Build history of the part. All positions in model axes, mm. A direction names the side the tool comes from. Give positions to 0.01 mm unless a question says otherwise; leave off trailing zeros. Order: outer loops, then holes, each group sorted by start corner. A loop starts at its lowest first (then second) coordinate and runs counter-clockwise, first axis right, second up. Notation, with made-up numbers: (38, -39.5) - (93, -39.5) arc R15 ccw to (93, -21.5) - close; hole circle Ø3 at (84, 55.5). An arc over 180 degrees is marked (long way). Use a Markdown table: item, result. Add a question column.
(1) Wall check: line 1 (Y direction, x = -8.5, z = 0); line 2 (Y direction, x = -14.55, z = 0); line 3 (Z direction, x = -7, y = -3.5). Give the ranges that are in metal, low to high.
(2) Slice it at A-A (y = 0). Write the cut outline in (x, z), then the cut area to 3 significant figures.
(3) Mould opens along Y. For faces 3 (the face through (-14.26, -15.62, -3.47)), 4 (the face through (0, -14, 14)), 5 (the face through (-6.844, -16.856, 8.767)), 6 (the face through (-7.409, -21.317, -2.799)) say: +Y half, -Y half, draft (parallel to the pull), parting line (faces both ways), or undercut.
(4) Slice it at C-C (x = -5.5). Write the cut outline in (y, z).
(5) Flat gauge pins, fed straight in: pin 1 (1.5 mm diameter, centred on x = -5.5, z = -14, fed in from -Y); pin 2 (5 mm diameter, centred on x = -5.5, z = 12.5, fed in from -Y); pin 3 (8 mm diameter, centred on y = 6.5, z = -7.5, fed in from -X); pin 4 (3 mm diameter, centred on x = -12.5, y = 5, fed in from +Z). Where does each tip first touch, or does it go through?
(6) Which spindle directions (+Z, -Z, +X, -X, +Y, -Y) get a long thin tool onto all of the face, cutting with end or side? Do faces 1 (the face through (-13.5, -13, -10)), 2 (the face through (-15, -11, 12)). Say none if no direction does.
Autodesk Inventor part; units mm, degrees
ref_plane "YZ Plane" through (0, 0, 0) normal (1, 0, 0) x (0, 1, 0)
ref_plane "XZ Plane" through (0, 0, 0) normal (0, 1, 0) x (-1, 0, 0)
ref_plane "XY Plane" through (0, 0, 0) normal (0, 0, 1) x (1, 0, 0)
sketch "Sketch1" plane through (0, 0, 0) normal (0, 1, 0) x (-1, 0, 0)
  line L0 (0, 0) -> (15, 0)
  line L1 (15, 16) -> (15, 21.5)
  line L2 (15, 21.5) -> (0, 21.5)
  line L3 (0, 21.5) -> (0, 19)
  line L4 (0, 19) -> (13.5, 19)
  line L5 (13.5, 19) -> (13.5, 16)
  line L6 (13.5, 16) -> (15, 16)
  dimension "d0" = 38
  dimension "d1" = 2.5
  dimension "d2" = 15
  dimension "d3" = 1.5
  dimension "d6" = 32
revolve "Revolution1" add sketch "Sketch1" angle 360 about axis through (0, 0, 0) along (-1, 0, 0)
chamfer "Chamfer1" distance 1 angle 45 2 edges at (0, 0, -21.5) (-15, 0, -21.5)
properties part number "031" material "Aluminum 6061"
Solution:
| question | item | result |
|---|---|---|
| 1 | line 1 | -21.5 to -19, 19 to 21.5 |
| 1 | line 2 | -20.95 to -16, 16 to 20.95 |
| 1 | line 3 | -21.21 to -18.67, 18.67 to 21.21 |
| 2 | outline | (-15, -20.5) - (-14, -21.5) - (-1, -21.5) - (0, -20.5) - (0, -19) - (-13.5, -19) - (-13.5, -16) - (-15, -16) - close; (-15, 16) - (-13.5, 16) - (-13.5, 19) - (0, 19) - (0, 20.5) - (-1, 21.5) - (-14, 21.5) - (-15, 20.5) - close |
| 2 | area | 82.0 mm2 |
| 3 | face 3 | undercut |
| 3 | face 4 | draft |
| 3 | face 5 | undercut |
| 3 | face 6 | parting line |
| 4 | outline | circle Ø43 at (0, 0); hole circle Ø38 at (0, 0) |
| 5 | pin 1 | y = -16.93 |
| 5 | pin 2 | y = -19.03 |
| 5 | pin 3 | through |
| 5 | pin 4 | z = 21.21 |
| 6 | face 1 | +X |
| 6 | face 2 | +Z, -Z, -X, +Y, -Y |
